Design review of the part built by this model. Coordinates are the model's own, in mm. A direction names the side the tool comes from. Coordinates: 2 decimals unless noted, no trailing zeros. Write each loop counter-clockwise with the first axis right and the second up, starting at its lowest first coordinate (ties: lowest second). Pieces come first, ordered by that corner, then holes.
```python
from build123d import *

# Parameters (mm, degrees)
F0_W     = 25.4
F0_H     = 25.4
F1_DEPTH = 203.2
F2_W     = 12.7
F2_H     = 12.7
F3_DEPTH = 12.7
F4_W     = 6.35
F4_H     = 12.7
F5_DEPTH = 12.7
F6_W     = 3.762882
F6_H     = 3.762882
F6_W_2   = 3.175
F6_H_2   = 3.175
F7_DEPTH = 177.8
F8_W     = 12.7
F8_H     = 12.7
F9_DEPTH = 25.4


with BuildPart() as f1:
    # F0 (on Top) → F1 (new body)
    with BuildSketch(Plane.XY):
        Rectangle(F0_W, F0_H)
    extrude(amount=F1_DEPTH)

    # F2 (on face) → F3 (join)
    with BuildSketch(Plane(origin=(0, 0, 0), x_dir=(1, 0, 0), z_dir=(0, 0, -1))):
        Rectangle(F2_W, F2_H)
    extrude(amount=F3_DEPTH)

    # F4 (on face) → F5 (cut)
    with BuildSketch(Plane(origin=(0, 0, -12.7), x_dir=(1, 0, 0), z_dir=(0, 0, -1))):
        with Locations((3.175, 0)):
            Rectangle(F4_W, F4_H)
    extrude(amount=-F5_DEPTH, mode=Mode.SUBTRACT)

    # F6 (on face) → F7 (cut)
    with BuildSketch(Plane.XY.offset(203.2)):
        with Locations((2.426788, 12.867747)):
            Rectangle(F6_W, F6_H)
        with Locations((-11.1125, 0)):
            Rectangle(F6_W_2, F6_H_2)
    extrude(amount=-F7_DEPTH, mode=Mode.SUBTRACT)

    # F8 (on face) → F9 (join)
    with BuildSketch(Plane.XY.offset(203.2)):
        Rectangle(F8_W, F8_H)
    extrude(amount=F9_DEPTH)


solid = f1.part
```
(1) Mouldability with a two-part tool opening along X and no side actions: class faces 5 (the flat face through (0, -6.35, 216)), 6 (the flat face through (-6.35, 0, -6)), 7 (the flat face through (2, 10.986, 116)) as +X half, -X half, draft (parallel to the pull), parting line (faces both ways), or undercut.
(2) Consider section A-A (z = 95). Give the boundary of the cut face in (x, y) (1 decimal), plus the area to 3 significant figures.
(3) Consider section B-B (x = -4). Give the boundary of the cut face in (y, z).
(4) Wall thickness on line 1 (Y direction, x = -11.5, z = 31); line 2 (Y direction, x = -1.25, z = 205); line 3 (Z direction, x = 6, y = -6.75): over which ranges is each line inside the solid? List them lowest first.
(5) For faces 1 (the flat face through (-3, -6.35, -6)), 2 (the flat face through (6.35, 0, 216)), 3 (the flat face through (0, 6.35, 216)), 4 (the flat face through (-6.35, 0, 216)), list the 3-axis set-ups (+Z, -Z, +X, -X, +Y, -Y) from which the entire face can be reached by the end or side of a thin tool; tool diameter is ignored.
(6) Consider section C-C (y = -8.5). Give the boundary of the cut face in (x, z).
(7) Insertion check: pin 1 Ø12 at (x, z) = (3, 124.5) entering from +Y; pin 2 Ø14 at (x, z) = (-2.5, 211) entering from -Y; pin 3 Ø10 at (x, z) = (-2, 218) entering from +Y; pin 4 Ø3.5 at (x, y) = (-10.5, 0) entering from +Z. Each pin has a flat end and moves straight along its axis. Give the tip position at first contact, or say it passes through.
Results:
1. face 5: draft
1. face 6: -X half
1. face 7: undercut
2. outline: (-12.7, -12.7) - (12.7, -12.7) - (12.7, 12.7) - (4.3, 12.7) - (4.3, 11) - (0.5, 11) - (0.5, 12.7) - (-12.7, 12.7) - (-12.7, 1.6) - (-9.5, 1.6) - (-9.5, -1.6) - (-12.7, -1.6) - close
2. area: 629 mm2
3. outline: (-12.7, 0) - (-6.35, 0) - (-6.35, -12.7) - (6.35, -12.7) - (6.35, 0) - (12.7, 0) - (12.7, 203.2) - (6.35, 203.2) - (6.35, 228.6) - (-6.35, 228.6) - (-6.35, 203.2) - (-12.7, 203.2) - close
4. line 1: y = -12.7 to -1.59, 1.59 to 12.7
4. line 2: y = -6.35 to 6.35
4. line 3: z = 0 to 203.2
5. face 1: -Z, +X, -X, -Y
5. face 2: +Z, +X, +Y, -Y
5. face 3: +Z, +X, -X, +Y
5. face 4: +Z, -X, +Y, -Y
6. outline: (-12.7, 0) - (12.7, 0) - (12.7, 203.2) - (-12.7, 203.2) - close
7. pin 1: stops at y = 12.7
7. pin 2: stops at y = -6.35
7. pin 3: stops at y = 6.35
7. pin 4: stops at z = 203.2
